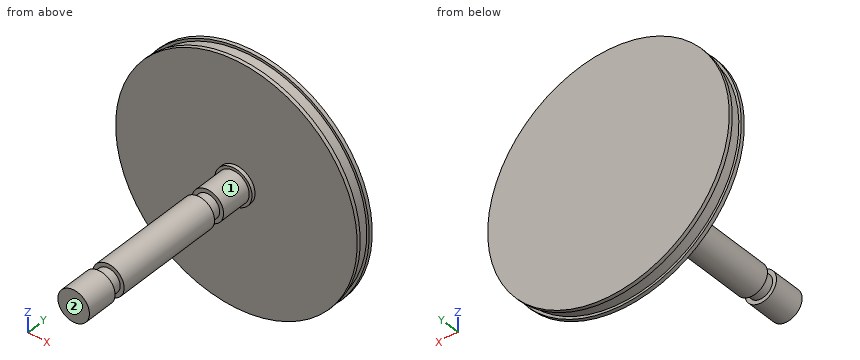
from build123d import *

# Parameters (mm, degrees)
SKETCH2_R           = 63.66
BOSS_EXTRUDE1_DEPTH = 5
SKETCH3_R           = 65
BOSS_EXTRUDE2_DEPTH = 2
SKETCH4_R           = 6.366
BOSS_EXTRUDE3_DEPTH = 108
SKETCH5_R           = 8.5
BOSS_EXTRUDE4_DEPTH = 17
SKETCH6_R           = 10
BOSS_EXTRUDE5_DEPTH = 2
BOSS_EXTRUDE6_START = 17
SKETCH7_R           = 8.5
BOSS_EXTRUDE6_DEPTH = 17
SKETCH8_R           = 8.5
BOSS_EXTRUDE7_DEPTH = 30


with BuildPart() as part:
    # Sketch2 → Boss-Extrude1 (new, symmetric)
    with BuildSketch(Plane(origin=(0, 0, 0), x_dir=(1, 0, 0), z_dir=(0, 1, 0))):
        with Locations(Location((0, 0, 0), (0, 0, 270))):
            Circle(SKETCH2_R)
    extrude(amount=BOSS_EXTRUDE1_DEPTH, both=True)

    # Sketch3 → Boss-Extrude2 (add)
    with BuildSketch(Plane.XZ.offset(5)):
        with Locations(Location((0, 0, 0), (0, 0, 270))):
            Circle(SKETCH3_R)
    boss_extrude2 = extrude(amount=-BOSS_EXTRUDE2_DEPTH)

    # Mirror1: Boss-Extrude2 across plane
    add(boss_extrude2.mirror(Plane.ZX))

    # Sketch4 → Boss-Extrude3 (add)
    with BuildSketch(Plane.XZ.offset(5)):
        with Locations(Location((0, 0, 0), (0, 0, 90))):
            Circle(SKETCH4_R)
    extrude(amount=BOSS_EXTRUDE3_DEPTH)

    # Sketch5 → Boss-Extrude4 (add)
    with BuildSketch(Plane.XZ.offset(113)):
        with Locations(Location((0, 0, 0), (0, 0, 270))):
            Circle(SKETCH5_R)
    extrude(amount=-BOSS_EXTRUDE4_DEPTH)

    # Sketch6 → Boss-Extrude5 (add)
    with BuildSketch(Plane.XZ.offset(5)):
        with Locations(Location((0, 0, 0), (0, 0, 90))):
            Circle(SKETCH6_R)
    extrude(amount=BOSS_EXTRUDE5_DEPTH)

    # Sketch7 → Boss-Extrude6 (add)
    with BuildSketch(Plane.XZ.offset(7).offset(BOSS_EXTRUDE6_START)):
        with Locations(Location((0, 0, 0), (0, 0, 270))):
            Circle(SKETCH7_R)
    extrude(amount=-BOSS_EXTRUDE6_DEPTH)

    # Sketch8 → Boss-Extrude7 (add, symmetric)
    with BuildSketch(Plane(origin=(0, -60, 0), x_dir=(-1, 0, 0), z_dir=(0, -1, 0))):
        with Locations(Location((0, 0, 0), (0, 0, 90))):
            Circle(SKETCH8_R)
    extrude(amount=BOSS_EXTRUDE7_DEPTH, both=True)


solid = part.part
Verification items for the finished model (mm, model axes). Face numbers are marked on the shaded views. A direction names the side the tool comes from. Round coordinates to 2 decimals unless told otherwise and drop trailing zeros. Loops run counter-clockwise (first coordinate to the right, second up) from the corner with the lowest first, then second, coordinate; pieces in that order, holes last. Notation, with made-up numbers: (-25.5, -19) - (-19.5, -19) arc R20 cw to (-19.5, 11) - close; hole circle Ø2 at (-34.5, 47). An arc over 180 degrees is marked (long way). Use a Markdown table: item, result. Add a question column.
1. Thickness scan on probe 1 along Y at (x, z) = (29, -4); probe 2 along Z at (x, y) = (1.5, -85); probe 3 along Z at (x, y) = (-25, -2.5). Record the ranges inside material, lowest first. Write a range as [from, to].
2. Access from +Z, -Z, +X, -X, +Y, -Y to the whole of each face (thin tool, end or side, straight path). Record for the marked faces 1 and 2.
3. Gauge pin test, flat ends, axial feed: pin 1 (4 mm diameter, centred on x = 18, z = 17.5, fed in from -Y); pin 2 (12 mm diameter, centred on y = -63.5, z = -2, fed in from +X). Record the tip position at first contact, or that the pin passes through.
4. Section check C-C, the plane z = 34.5. Record the boundary of the cut face in (x, y).
5. Section check B-B, the plane y = -87.5. Record the boundary of the cut face in (x, z), plus the area to 3 significant figures.
6. Section check A-A, the plane z = 12. Record the boundary of the cut face in (x, y).
Checks:
| question | item | result |
|---|---|---|
| 1 | probe 1 | y = [-5, 5] |
| 1 | probe 2 | z = [-8.37, 8.37] |
| 1 | probe 3 | z = [-58.55, 58.55] |
| 2 | face 1 | -Y |
| 2 | face 2 | +Z, -Z, +X, -X, -Y |
| 3 | pin 1 | stops at y = -5 |
| 3 | pin 2 | stops at x = 8.5 |
| 4 | outline | (-55.09, -5) - (55.09, -5) - (55.09, -3) - (53.5, -3) - (53.5, 3) - (55.09, 3) - (55.09, 5) - (-55.09, 5) - (-55.09, 3) - (-53.5, 3) - (-53.5, -3) - (-55.09, -3) - close |
| 5 | outline | circle Ø17 at (0, 0) |
| 5 | area | 227 mm^2 |
| 6 | outline | (-63.88, -5) - (63.88, -5) - (63.88, -3) - (62.52, -3) - (62.52, 3) - (63.88, 3) - (63.88, 5) - (-63.88, 5) - (-63.88, 3) - (-62.52, 3) - (-62.52, -3) - (-63.88, -3) - close |
